Could you check a few things on this model? Use its own coordinates, in mm. A direction names the side the tool comes from. Give positions to 0.01 mm unless a question says otherwise; leave off trailing zeros. Loops run counter-clockwise (first coordinate to the right, second up) from the corner with the lowest first, then second, coordinate; pieces in that order, holes last. Notation, with made-up numbers: M -6,-15.5 L 52,-15.5 A31 cw 52,10.5 Z; hole C 40.25,57 d7. An arc over 180 degrees is marked long. Answer in a Markdown table with one row per item. Add a question column.
```python
from build123d import *

# Parameters (mm, degrees)
SKETCH_W        = 10.1
SKETCH_H        = 7.1
PAD_DEPTH       = 1
SKETCH001_W     = 10
SKETCH001_H     = 7
PAD001_DEPTH    = 15
POCKET_DEPTH    = 7.051
SKETCH003_W     = 6
SKETCH003_H     = 4
POCKET001_DEPTH = 8


with BuildPart() as part:
    # Sketch → Pad (new body)
    with BuildSketch(Plane.XY):
        Rectangle(SKETCH_W, SKETCH_H)
    extrude(amount=PAD_DEPTH)

    # Sketch001 → Pad001 (new body)
    with BuildSketch(Plane.XY.offset(1)):
        Rectangle(SKETCH001_W, SKETCH001_H)
    extrude(amount=PAD001_DEPTH)

    # Sketch002 → Pocket (cut, through all)
    with BuildSketch(Plane.XZ.offset(3.5)):
        Polygon((5, 16), (-20, 16), (-20, -4), align=None)
    extrude(amount=-POCKET_DEPTH, mode=Mode.SUBTRACT)

    # Sketch003 → Pocket001 (cut)
    with BuildSketch(Plane(origin=(0, 0, 0), x_dir=(1, 0, 0), z_dir=(0, 0, -1))):
        Rectangle(SKETCH003_W, SKETCH003_H)
    extrude(amount=-POCKET001_DEPTH, mode=Mode.SUBTRACT)


solid = part.part
```
Item 1: Suppose I cut it at B-B (x = 1.5). List the corners of the cut face in (y, z) for me, then the cut area to 3 significant figures.
Item 2: If we mould it in two halves opening along X, with no side actions, what happens to faces 5 (the face through (5.05, 0, 0.5)), 6 (the face through (-3, 0, 4)), 7 (the face through (-5.05, 0, 0.5))? For each: +X half, -X half, draft (parallel to the pull), parting line (faces both ways), or undercut.
Item 3: For P1, Ø5, axis at x = -2, z = 10.5, coming from the +Y side; P2, Ø1.5, axis at y = 0.5, z = 6.5, coming from the +X side; P3, Ø1, axis at y = 0.5, z = 12, coming from the -X side (3 decimals), each with a flat end and sliding along its axis, tell me the tip position at first contact or that it passes through.
Item 4: Suppose I cut it at A-A (y = -2.5). List the corners of the cut face in (x, z) for me, then the cut area to 3 significant figures.
Item 5: I need wall thicknesses on L1, parallel to Y at x = -0.5, z = 7; L2, parallel to X at y = 1.25, z = 3.75; L3, parallel to Y at x = -0.75, z = 10.5. Which ranges of each line are inside material? Lowest first, please.
Item 6: For faces 1 (the face through (5, 0, 8)), 2 (the face through (-5, 0, 4)), 3 (the face through (1, 3.5, 7)), 4 (the face through (3, 0, 4)), which set-ups out of +Z, -Z, +X, -X, +Y, -Y let a thin tool reach every point of the face, with its end or its side?
Item 7: Suppose I cut it at C-C (z = 5.5). List the corners of the cut face in (x, y) for me, then the cut area to 3 significant figures.
Item 8: Suppose I cut it at D-D (y = 1.25). List the corners of the cut face in (x, z) for me, then the cut area to 3 significant figures.
Values found:
| question | item | result |
|---|---|---|
| 1 | outline | M -3.55,0 L -2,0 L -2,8 L 2,8 L 2,0 L 3.55,0 L 3.55,1 L 3.5,1 L 3.5,13.2 L -3.5,13.2 L -3.5,1 L -3.55,1 Z |
| 1 | area | 60.5 mm² |
| 2 | face 5 | +X half |
| 2 | face 6 | undercut |
| 2 | face 7 | -X half |
| 3 | P1 | y = 3.5 |
| 3 | P2 | x = 5 |
| 3 | P3 | x = -0.625 |
| 4 | outline | M -5.05,0 L 5.05,0 L 5.05,1 L 5,1 L 5,16 L -5,8 L -5,1 L -5.05,1 Z |
| 4 | area | 120 mm² |
| 5 | L1 | -3.5 to -2, 2 to 3.5 |
| 5 | L2 | -5 to -3, 3 to 5 |
| 5 | L3 | -3.5 to 3.5 |
| 6 | face 1 | +Z, +X, +Y, -Y |
| 6 | face 2 | +Z, -X, +Y, -Y |
| 6 | face 3 | +Z, +X, -X, +Y |
| 6 | face 4 | -Z |
| 7 | outline | M -5,-3.5 L 5,-3.5 L 5,3.5 L -5,3.5 Z; hole M -3,-2 L 3,-2 L 3,2 L -3,2 Z |
| 7 | area | 46.0 mm² |
| 8 | outline | M -5.05,0 L -3,0 L -3,8 L 3,8 L 3,0 L 5.05,0 L 5.05,1 L 5,1 L 5,16 L -5,8 L -5,1 L -5.05,1 Z |
| 8 | area | 72.1 mm² |
